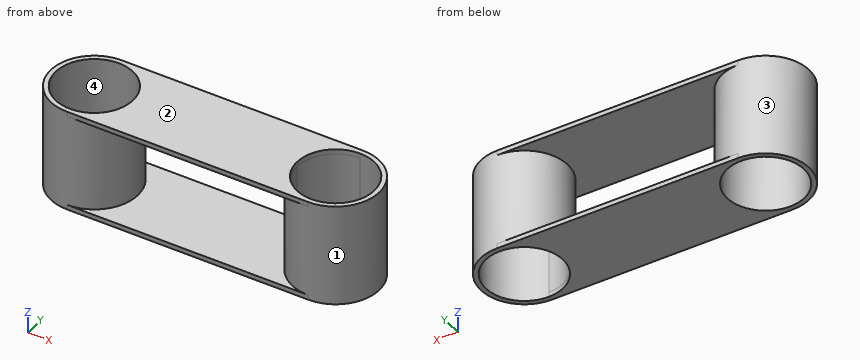
```python
from build123d import *

# Parameters (mm, degrees)
SKETCH1_R               = 90
SKETCH1_R_2             = 80
BOSS_EXTRUDE1_DEPTH     = 106
BOSS_EXTRUDE2_DEPTH     = 10
CUT_EXTRUDE1_DEPTH      = 631.082534276
CUT_EXTRUDE1_DEPTH_BACK = 631.082534276


with BuildPart() as part:
    # Sketch1 → Boss-Extrude1 (new, symmetric)
    with BuildSketch(Plane.XY):
        Circle(SKETCH1_R)
        Circle(SKETCH1_R_2, mode=Mode.SUBTRACT)
    boss_extrude1 = extrude(amount=BOSS_EXTRUDE1_DEPTH, both=True)

    # Sketch2 → Boss-Extrude2 (add)
    with BuildSketch(Plane.XY.offset(106)):
        with BuildLine():
            Line((0, 90), (499.88, 90))
            Line((499.88, 90), (499.88, -90))
            Line((499.88, -90), (0, -90))
            ThreePointArc((0, -90), (90, 0), (0, 90))
        make_face()
    boss_extrude2 = extrude(amount=-BOSS_EXTRUDE2_DEPTH)

    # Mirror1: Boss-Extrude2 across plane
    add(boss_extrude2.mirror(Plane.XY))

    # Mirror2: Boss-Extrude1 across plane
    add(boss_extrude1.mirror(Plane(origin=(250, 0, 0), x_dir=(0, 0, 1), z_dir=(1, 0, 0))))

    # Sketch3 → Cut-Extrude1 (cut, two sides: drawn at the far end of the back side and taken through both)
    with BuildSketch(Plane.XY.offset(-96).offset(-CUT_EXTRUDE1_DEPTH_BACK)):
        with BuildLine():
            Line((499.88, -79.99991), (499.88, 79.99991))
            ThreePointArc((499.88, 79.99991), (420, 0), (499.88, -79.99991))
        make_face()
    extrude(amount=CUT_EXTRUDE1_DEPTH + CUT_EXTRUDE1_DEPTH_BACK, mode=Mode.SUBTRACT)


solid = part.part
```
Verification items for the finished model (mm, model axes). Face numbers are marked on the shaded views. A direction names the side the tool comes from. Round coordinates to 2 decimals unless told otherwise and drop trailing zeros. Write each loop counter-clockwise with the first axis right and the second up, starting at its lowest first coordinate (ties: lowest second). Pieces come first, ordered by that corner, then holes. Notation, with made-up numbers: (-9, 4.5) -> (-5, 4.5) arc R23 ccw to (-5, 17.5) -> close; hole circle Ø4 at (87.5, 14). An arc over 180 degrees is marked (long way). Write each question's results on one line, items separated by ' | '.
Q1. Sectioned sample at C-C, the plane z = 64. Record the boundary of the cut face in (x, y), and give its area (3 significant figures).
Derived:
outline: circle Ø180 at (0, 0); circle Ø180 at (500, 0); hole circle Ø160 at (0, 0); hole circle Ø160 at (500, 0) | area: 10,700 mm²
Q2. Sectioned sample at A-A, the plane x = 201.5. Record the boundary of the cut face in (y, z).
Derived:
outline: (-90, -106) -> (90, -106) -> (90, -96) -> (-90, -96) -> close; (-90, 96) -> (90, 96) -> (90, 106) -> (-90, 106) -> close
Q3. Go/stop test with flat-tipped pins: pin 1 Ø12 at (y, z) = (31, 69) entering from -X; pin 2 Ø2 at (y, z) = (-16.5, -50) entering from -X; pin 3 Ø2 at (x, z) = (34.5, -73) entering from +Y. Record where each tip stops, or that it passes through.
Derived:
pin 1: stops at x = -86.46 | pin 2: stops at x = -88.66 | pin 3: stops at y = 83.53
Q4. Thickness scan on probe 1 along Z at (x, y) = (144, 32); probe 2 along X at (y, z) = (66, -18); probe 3 along X at (y, z) = (-26, 10). Record the ranges inside material, lowest first.
Derived:
probe 1: z = -106 to -96, 96 to 106 | probe 2: x = -61.19 to -45.21, 45.21 to 61.19, 438.81 to 454.79, 545.21 to 561.19 | probe 3: x = -86.16 to -75.66, 75.66 to 86.16, 413.84 to 424.34, 575.66 to 586.16
Q5. Draft check along X on the marked faces 1 and 2. Enter one of: released by +X, released by -X, zero draft, split by the parting line, or undercut.
Derived:
face 1: undercut | face 2: zero draft
Q6. Access from +Z, -Z, +X, -X, +Y, -Y to the whole of each face (thin tool, end or side, straight path). Record for the marked faces 3 and 4.
Derived:
face 3: none | face 4: +Z, -Z
Q7. Sectioned sample at D-D, the plane x = 510. Record the boundary of the cut face in (y, z).
Derived:
outline: (-89.44, -106) -> (-79.37, -106) -> (-79.37, 106) -> (-89.44, 106) -> close; (79.37, -106) -> (89.44, -106) -> (89.44, 106) -> (79.37, 106) -> close
Q8. Sectioned sample at B-B, the plane y = -45. Record the boundary of the cut face in (x, z).
Derived:
outline: (-77.94, -106) -> (-66.14, -106) -> (-66.14, 106) -> (-77.94, 106) -> close; (66.14, -106) -> (433.86, -106) -> (433.86, 106) -> (66.14, 106) -> close; (566.14, -106) -> (577.94, -106) -> (577.94, 106) -> (566.14, 106) -> close; hole (77.94, -96) -> (422.06, -96) -> (422.06, 96) -> (77.94, 96) -> close
